Drawing for the job (mm, zero at the part's lowest x, y, z). Coordinates: 2 decimals unless noted, no trailing zeros. Order: outer loops, then holes, each group sorted by start corner. A loop starts at its lowest first (then second) coordinate and runs counter-clockwise, first axis right, second up.
1) Pin check, flat tips, straight feed: pin 1 Ø12 at (x, y) = (12, 27) entering from +Z (1 decimal); pin 2 Ø1.5 at (y, z) = (30.5, 5) entering from +X (1 decimal); pin 3 Ø1.5 at (x, z) = (18.04, 15.11) entering from +Y; pin 4 Ø1.5 at (x, y) = (15.5, 39.5) entering from +Z. Stop position of each tip, or through.
2) Cut at D-D (x = 8). List the corners of the cut face in (y, z) (1 decimal).
3) Wall check: L1, parallel to Z at x = 12, y = 27.5 (1 decimal); L2, parallel to Z at x = 3.25, y = 29 (1 decimal); L3, parallel to X at y = 24, z = 11 (1 decimal). Give the ranges that are in metal, low to high.
4) Cut at C-C (x = 18). List the corners of the cut face in (y, z), and give its area (3 significant figures).
5) Cut at B-B (x = 3.5). List the corners of the cut face in (y, z).
6) Cut at A-A (y = 36.5). Give the number of separate pieces and of enclosed holes in the cut face.
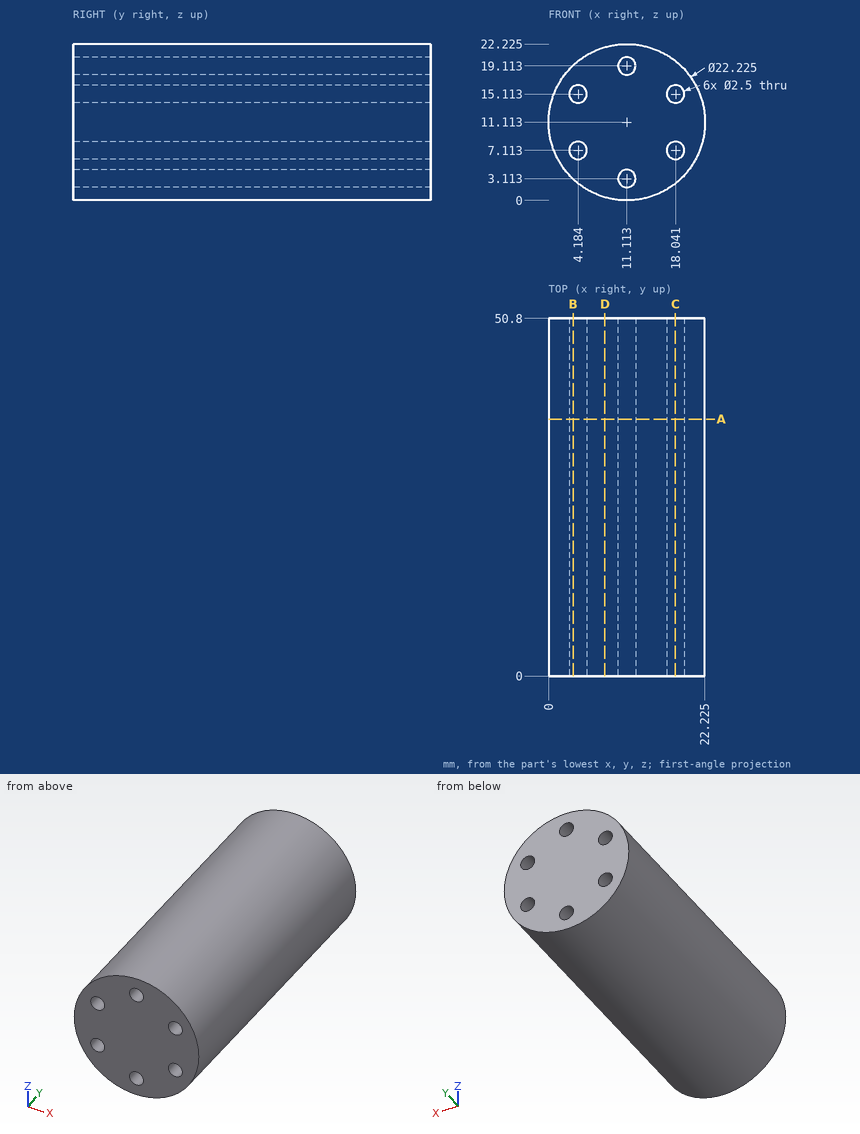
Geometry check:
1. pin 1: stops at z = 22.2
1. pin 2: stops at x = 20.8
1. pin 3: passes through
1. pin 4: stops at z = 21.61
2. outline: (0, 0.4) - (50.8, 0.4) - (50.8, 21.8) - (0, 21.8) - close
3. L1: z = 0 to 2.2, 4 to 18.2, 20 to 22.2
3. L2: z = 3.3 to 6.3, 7.9 to 14.3, 15.9 to 19
3. L3: x = 0 to 22.2
4. outline: (0, 2.39) - (50.8, 2.39) - (50.8, 5.86) - (0, 5.86) - close; (0, 8.36) - (50.8, 8.36) - (50.8, 13.86) - (0, 13.86) - close; (0, 16.36) - (50.8, 16.36) - (50.8, 19.83) - (0, 19.83) - close
4. area: 632 mm2
5. outline: (0, 3.02) - (50.8, 3.02) - (50.8, 6.07) - (0, 6.07) - close; (0, 8.16) - (50.8, 8.16) - (50.8, 14.07) - (0, 14.07) - close; (0, 16.16) - (50.8, 16.16) - (50.8, 19.21) - (0, 19.21) - close
6. separate pieces: 1
6. enclosed holes: 6
